Autodesk Inventor part; units mm, degrees
ref_plane "YZ Plane" through (0, 0, 0) normal (1, 0, 0) x (0, 1, 0)
ref_plane "XZ Plane" through (0, 0, 0) normal (0, 1, 0) x (-1, 0, 0)
ref_plane "XY Plane" through (0, 0, 0) normal (0, 0, 1) x (1, 0, 0)
sketch "Skizze1" plane through (0, 0, 0) normal (0, 0, 1) x (1, 0, 0)
  circle A0 centre (0, 0) radius 4
  dimension "d0" = 8
extrude "Extrusion1" add sketch "Skizze1" along normal blind 10
sketch "Skizze2" plane through (0, 0, 10) normal (0, 0, 1) x (1, 0, 0)
  circle A0 centre (0, 0) radius 3.5
  dimension "d3" = 7
extrude "Extrusion2" cut sketch "Skizze2" against normal blind 9
sketch "Skizze3" plane through (0, 0, 10) normal (0, 0, 1) x (1, 0, 0)
  circle A0 centre (0, 0) radius 3.5
extrude "Extrusion3" add sketch "Skizze3" against normal blind 1
sketch "Skizze4" plane through (0, 0, 10) normal (0, 0, 1) x (1, 0, 0)
  circle A0 centre (0, 0) radius 0.5
  dimension "d8" = 1
extrude "Extrusion4" cut sketch "Skizze4" against normal blind 1
sketch "Skizze5" plane through (0, 0, 10) normal (0, 0, 1) x (1, 0, 0)
  circle A0 centre (-2.5, 0) radius 0.5
  circle A1 centre (0, 0) radius 4
  line L0 (-5.6, 0) -> (5.6, 0)
  dimension "d11" = 1
  dimension "d12" = 2.5
  dimension "d13" = 0
extrude "Extrusion5" cut sketch "Skizze5" against normal blind 1 contours L0 A0 | A0 L0
sketch "Skizze6" plane through (0, 0, 0) normal (0, 0, -1) x (-1, 0, 0)
  circle A0 centre (2.5, 0) radius 0.5
  line L0 (5.6, 0) -> (-5.6, 0)
  point P0 (0, 0)
  dimension "d16" = 1
  dimension "d17" = 2.5
  dimension "d18" = 0
extrude "Extrusion6" cut sketch "Skizze6" against normal blind 1
properties part number "Pneumatickolben_Zylinder"
The model under review builds one solid part; all positions refer to its coordinate system, in mm. A direction names the side the tool comes from. Coordinates: 2 decimals unless noted, no trailing zeros. Order: outer loops, then holes, each group sorted by start corner. A loop starts at its lowest first (then second) coordinate and runs counter-clockwise, first axis right, second up. Notation, with made-up numbers: (59, 64) -> (67, 64) arc R28 ccw to (67, 92) -> close; hole circle Ø6 at (21, 23.5). An arc over 180 degrees is marked (long way). Answer in a Markdown table with one row per item.
(1) The part is to be moulded in two halves that separate along X. For faces 4 (the cylindrical face through (-0.867, 3.905, 4.93)), 5 (the flat face through (0, 0, 0)), 6 (the cylindrical face through (-2.9, -0.3, 9.5)), say which applies: +X half, -X half, draft (parallel to the pull), parting line (faces both ways), or undercut.
Answers:
| item | result |
|---|---|
| face 4 | parting line |
| face 5 | draft |
| face 6 | undercut |
(2) Consider section B-B (x = -1.75). Write out the cut boundary in (y, z).
Answers:
| item | result |
|---|---|
| outline | (-3.6, 0) -> (3.6, 0) -> (3.6, 10) -> (-3.6, 10) -> close; hole (-3.03, 1) -> (3.03, 1) -> (3.03, 9) -> (-3.03, 9) -> close |
(3) Wall thickness on line 1 along Z through (x, y) = (-1.25, -1.75); line 2 along Y through (x, z) = (0, 9.8); line 3 along Y through (x, z) = (0, 5.75): over which ranges is each line inside the solid? List them lowest first.
Answers:
| item | result |
|---|---|
| line 1 | 0 to 1, 9 to 10 |
| line 2 | -4 to -0.5, 0.5 to 4 |
| line 3 | -4 to -3.5, 3.5 to 4 |
(4) Machinability: for faces 1 (the flat face through (0, 0, 1)), 2 (the flat face through (1, 0, 10)), 3 (the cylindrical face through (-0.108, -0.488, 9.507)), which of the approach directions +Z, -Z, +X, -X, +Y, -Y give a long, thin tool a straight path to every point of the face, cutting with its end or side? Answer none if there is none.
Answers:
| item | result |
|---|---|
| face 1 | none |
| face 2 | +Z, +X, -X, +Y, -Y |
| face 3 | +Z |
(5) Consider section C-C (x = 0). Write out the cut boundary in (y, z).
Answers:
| item | result |
|---|---|
| outline | (-4, 0) -> (4, 0) -> (4, 10) -> (0.5, 10) -> (0.5, 9) -> (3.5, 9) -> (3.5, 1) -> (-3.5, 1) -> (-3.5, 9) -> (-0.5, 9) -> (-0.5, 10) -> (-4, 10) -> close |
(6) Insertion check: pin 1 (1.5 mm diameter, centred on y = -3, z = 5.5, fed in from -X); pin 2 (3 mm diameter, centred on x = -3, z = 9, fed in from -Y). Each pin has a flat end and moves straight along its axis. Give the tip position at first contact, or say it passes through.
Answers:
| item | result |
|---|---|
| pin 1 | x = -3.31 |
| pin 2 | y = -3.71 |
(7) Consider section D-D (y = 3). Write out the cut boundary in (x, z), plus the area to 3 significant figures.
Answers:
| item | result |
|---|---|
| outline | (-2.65, 0) -> (2.65, 0) -> (2.65, 10) -> (-2.65, 10) -> close; hole (-1.8, 1) -> (1.8, 1) -> (1.8, 9) -> (-1.8, 9) -> close |
| area | 24.1 mm² |
(8) Consider section A-A (y = 0). Write out the cut boundary in (x, z).
Answers:
| item | result |
|---|---|
| outline | (-4, 0) -> (-3, 0) -> (-3, 1) -> (-3.5, 1) -> (-3.5, 9) -> (-3, 9) -> (-3, 10) -> (-4, 10) -> close; (-2, 0) -> (4, 0) -> (4, 10) -> (0.5, 10) -> (0.5, 9) -> (3.5, 9) -> (3.5, 1) -> (-2, 1) -> close; (-2, 9) -> (-0.5, 9) -> (-0.5, 10) -> (-2, 10) -> close |
